from build123d import *

# Parameters (mm, degrees)
BOX027_W     = 77
BOX027_H     = 2
BOX027_DEPTH = 100.5
FILLET031_R  = 10
BOX026_W     = 80
BOX026_H     = 2
BOX026_DEPTH = 103.5
FILLET030_R  = 10
FILLET032_R  = 0.25


with BuildPart() as obj1:
    # Box027 → Box027 (new body)
    with BuildSketch(Plane(origin=(0.5, -26, -13.25), x_dir=(1, 0, 0), z_dir=(0, 0, 1))):
        with Locations((38.5, 1)):
            Rectangle(BOX027_W, BOX027_H)
    extrude(amount=BOX027_DEPTH)

    # Fillet031
    fillet031_edges = [obj1.edges().sort_by_distance(p)[0] for p in [
        (0.5, -25, 87.25),
        (0.5, -25, -13.25),
        (77.5, -25, 87.25),
        (77.5, -25, -13.25),
    ]]
    fillet(fillet031_edges, radius=FILLET031_R)


with BuildPart() as obj1_1:
    # Fillet031 placement: moved
    add(obj1.part.moved(Location((0, 0.5, 0))))


with BuildPart() as ridge:
    # Box026 → Box026 (new body)
    with BuildSketch(Plane(origin=(-1, -26, -14.75), x_dir=(1, 0, 0), z_dir=(0, 0, 1))):
        with Locations((40, 1)):
            Rectangle(BOX026_W, BOX026_H)
    extrude(amount=BOX026_DEPTH)

    # Fillet030
    fillet030_edges = [ridge.edges().sort_by_distance(p)[0] for p in [
        (-1, -25, 88.75),
        (-1, -25, -14.75),
        (79, -25, 88.75),
        (79, -25, -14.75),
    ]]
    fillet(fillet030_edges, radius=FILLET030_R)


with BuildPart() as ridge_1:
    # Fillet030 placement: moved
    add(ridge.part.moved(Location((0, 0.5, 0))))

    # Cut008: cut obj1
    add(obj1_1.part, mode=Mode.SUBTRACT)

    # Fillet032
    fillet032_edges = [ridge_1.edges().sort_by_distance(p)[0] for p in [
        (-1, -23.5, 37),
        (1.928932, -23.5, -11.821068),
        (39, -23.5, -14.75),
        (76.071068, -23.5, -11.821068),
        (79, -23.5, 37),
        (1.928932, -23.5, 85.821068),
        (76.071068, -23.5, 85.821068),
        (39, -23.5, 88.75),
        (0.5, -23.5, 37),
        (3.428932, -23.5, 84.321068),
        (39, -23.5, 87.25),
        (74.571068, -23.5, 84.321068),
        (77.5, -23.5, 37),
        (74.571068, -23.5, -10.321068),
        (39, -23.5, -13.25),
        (3.428932, -23.5, -10.321068),
    ]]
    fillet(fillet032_edges, radius=FILLET032_R)


solid = ridge_1.part
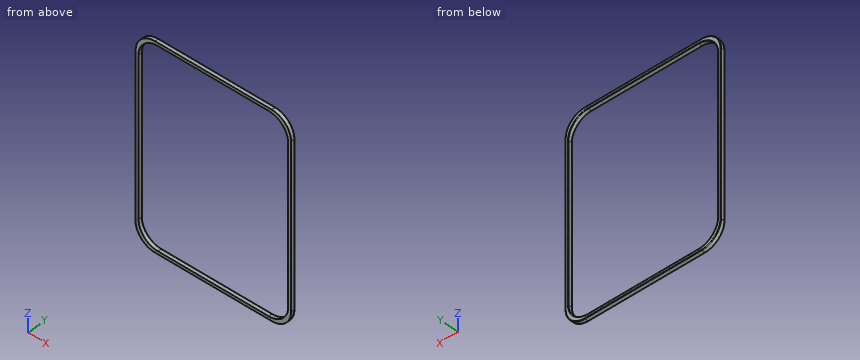
Can you work these out from the model? Positions are in its coordinate system, mm. Give positions to 0.01 mm unless a question says otherwise; leave off trailing zeros. Write each loop counter-clockwise with the first axis right and the second up, starting at its lowest first coordinate (ties: lowest second). Pieces come first, ordered by that corner, then holes. Notation, with made-up numbers: M 57,56 L 85,56 A20 cw 85,84 Z; hole C 73.25,21 d4. An arc over 180 degrees is marked long. Answer in a Markdown table with one row per item. Add a question column.
Item 1: Imagine slicing it at A-A, the plane z = 31.5. Write out the boundary of the cut face in (x, y), plus the area to 3 significant figures.
Item 2: Imagine slicing it at C-C, the plane y = -24.6. Write out the boundary of the cut face in (x, z), plus the area to 4 significant figures.
Item 3: Imagine slicing it at B-B, the plane x = 34.5. Write out the boundary of the cut face in (y, z).
Item 4: Please list where these lines run through material, in increasing order: L1, parallel to X at y = -25.15, z = 49.5; L2, parallel to Z at x = 44.5, y = -24.45; L3, parallel to Z at x = 56, y = -23.7.
Evaluation:
| question | item | result |
|---|---|---|
| 1 | outline | M -1,-25.5 L 0.5,-25.5 L 0.5,-23.75 A0.25 ccw 0.25,-23.5 L -0.75,-23.5 A0.25 ccw -1,-23.75 Z; M 77.5,-25.5 L 79,-25.5 L 79,-23.75 A0.25 ccw 78.75,-23.5 L 77.75,-23.5 A0.25 ccw 77.5,-23.75 Z |
| 1 | area | 5.95 mm² |
| 2 | outline | M -1,-4.75 A10 ccw 9,-14.75 L 69,-14.75 A10 ccw 79,-4.75 L 79,78.75 A10 ccw 69,88.75 L 9,88.75 A10 ccw -1,78.75 Z; hole M 0.5,-3.25 A10 ccw 10.5,-13.25 L 67.5,-13.25 A10 ccw 77.5,-3.25 L 77.5,77.25 A10 ccw 67.5,87.25 L 10.5,87.25 A10 ccw 0.5,77.25 Z |
| 2 | area | 541.5 mm² |
| 3 | outline | M -25.5,-14.75 L -23.75,-14.75 A0.25 ccw -23.5,-14.5 L -23.5,-13.5 A0.25 ccw -23.75,-13.25 L -25.5,-13.25 Z; M -25.5,87.25 L -23.75,87.25 A0.25 ccw -23.5,87.5 L -23.5,88.5 A0.25 ccw -23.75,88.75 L -25.5,88.75 Z |
| 4 | L1 | x = -1 to 0.5, 77.5 to 79 |
| 4 | L2 | z = -14.75 to -13.25, 87.25 to 88.75 |
| 4 | L3 | z = -14.74 to -13.26, 87.26 to 88.74 |
